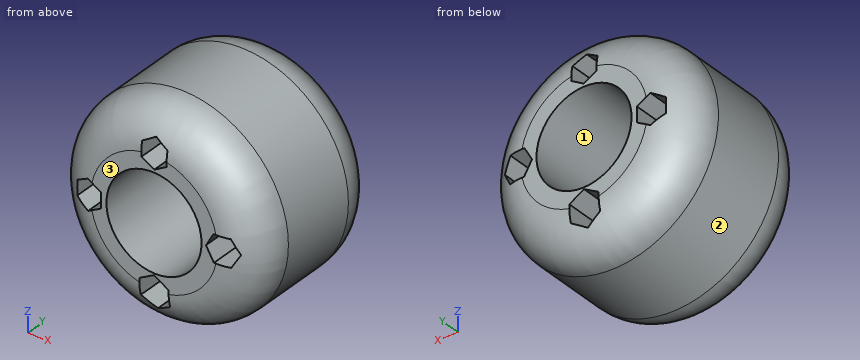
```python
from build123d import *

# Parameters (mm, degrees)
F0_R     = 5
F0_R_2   = 2.3
F1_DEPTH = 3.8


# Not quite as in the source:
# - a fillet or chamfer that OpenCascade refuses, or shapes differently, is made with other operations: its cross-section is extruded or revolved along the edge and cut away or added


with BuildPart() as f1:
    # F0 (on Front) → F1 (new body, symmetric)
    with BuildSketch(Plane.XZ):
        Circle(F0_R)
        Polygon((0, -4.0174636819), (-0.7082950324, -3.6085293543), (-0.7082950324, -2.7906606991), (0, -2.3817263714), (0.7082950324, -2.7906606991), (0.7082950324, -3.6085293543), align=None, mode=Mode.SUBTRACT)
        Polygon((-3.1964122335, 0.7368465077), (-2.5582844391, 0.3684232539), (-2.5582844391, -0.3684232539), (-3.1964122335, -0.7368465077), (-3.8345400279, -0.3684232539), (-3.8345400279, 0.3684232539), align=None, mode=Mode.SUBTRACT)
        Circle(F0_R_2, mode=Mode.SUBTRACT)
        Polygon((2.8982667587, -0.6579181574), (2.512562897, -0.0101405277), (2.8807028495, 0.6477776297), (3.6345466637, 0.6579181574), (4.0202505254, 0.0101405277), (3.6521105729, -0.6477776297), align=None, mode=Mode.SUBTRACT)
        Polygon((0.6046901305, 3.5066245139), (0.6168706685, 2.8013560578), (0.012180538, 2.4381731744), (-0.6046901305, 2.7802587472), (-0.6168706685, 3.4855272032), (-0.012180538, 3.8487100866), align=None, mode=Mode.SUBTRACT)
    extrude(amount=F1_DEPTH, both=True)

    # F2: fillet of radius 1.9313708499 on 3 edges, made by hand

    # F2_s1 → F2_t2 (revolve, cut)
    with BuildSketch(Plane.XY):
        with BuildLine():
            ThreePointArc((5, 1.8686291501), (4.4343145751, 3.2343145751), (3.0686291501, 3.8))
            Line((3.0686291501, 3.8), (5, 3.8))
            Line((5, 3.8), (5, 1.8686291501))
        make_face()
    revolve(axis=Axis((0, 3.8, 0), (0, -1, 0)), mode=Mode.SUBTRACT)

    # F2_s3 → F2_t4 (revolve, cut)
    with BuildSketch(Plane.XY):
        with BuildLine():
            ThreePointArc((5, -1.8686291501), (4.4343145751, -3.2343145751), (3.0686291501, -3.8))
            Line((3.0686291501, -3.8), (5, -3.8))
            Line((5, -3.8), (5, -1.8686291501))
        make_face()
    revolve(axis=Axis((0, -3.8, 0), (0, -1, 0)), mode=Mode.SUBTRACT)


solid = f1.part
```
Work out the finished part from the listing and answer in its coordinate system (mm). Face numbers are marked on the shaded views. Round coordinates to 2 decimals unless told otherwise and drop trailing zeros. Loops run counter-clockwise (first coordinate to the right, second up) from the corner with the lowest first, then second, coordinate; pieces in that order, holes last.
(1) Each of these flat-tipped pins is pushed along its axis until it touches: P1, Ø5, axis at x = 2, z = -3.5, coming from the +Y side; P2, Ø3, axis at y = 0.5, z = -3, coming from the +X side; P3, Ø2, axis at y = 2, z = -2.5, coming from the -X side; P4, Ø0.9, axis at y = -0.5, z = -3, coming from the -X side. Where does it stop, or does it pass through?
Computed values:
P1: stops at y = 3.8
P2: stops at x = 4.77
P3: stops at x = -4.77
P4: stops at x = -4.3
(2) The mould has two halves that part along X. Classify the marked faces 1, 2 and 3: pulls with the +X half, pulls with the -X half, needs draft (parallel to the pull), parting line crosses it, or undercut.
Computed values:
face 1: undercut
face 2: parting line crosses it
face 3: needs draft
(3) Find the intervals of material crossed by L1, parallel to Z at x = 1.5, y = 2.75; L2, parallel to Z at x = -3.5, y = -0.75; L3, parallel to Y at x = -2.75, z = 2.25, in increasing order.
Computed values:
L1: z = -4.55 to -1.74, 1.74 to 4.55
L2: z = -3.57 to -0.56, 0.56 to 3.57
L3: y = -3.74 to 3.74
(4) The part is cut by section B-B, the plane y = -3. Give the vertices of the cut face in (x, z), and give its area (3 significant figures).
Computed values:
outline: circle Ø9.27 at (0, 0); hole (-3.83, -0.37) - (-3.2, -0.74) - (-2.56, -0.37) - (-2.56, 0.37) - (-3.2, 0.74) - (-3.83, 0.37) - close; hole circle Ø4.6 at (0, 0); hole (-0.71, -3.61) - (0, -4.02) - (0.71, -3.61) - (0.71, -2.79) - (0, -2.38) - (-0.71, -2.79) - close; hole (-0.62, 3.49) - (-0.6, 2.78) - (0.01, 2.44) - (0.62, 2.8) - (0.6, 3.51) - (-0.01, 3.85) - close; hole (2.51, -0.01) - (2.9, -0.66) - (3.65, -0.65) - (4.02, 0.01) - (3.63, 0.66) - (2.88, 0.65) - close
area: 44.9 mm2
(5) The part is cut by section A-A, the plane y = 1. Give the vertices of the cut face in (x, z), and give its area (3 significant figures).
Computed values:
outline: circle Ø10 at (0, 0); hole (-3.83, -0.37) - (-3.2, -0.74) - (-2.56, -0.37) - (-2.56, 0.37) - (-3.2, 0.74) - (-3.83, 0.37) - close; hole circle Ø4.6 at (0, 0); hole (-0.71, -3.61) - (0, -4.02) - (0.71, -3.61) - (0.71, -2.79) - (0, -2.38) - (-0.71, -2.79) - close; hole (-0.62, 3.49) - (-0.6, 2.78) - (0.01, 2.44) - (0.62, 2.8) - (0.6, 3.51) - (-0.01, 3.85) - close; hole (2.51, -0.01) - (2.9, -0.66) - (3.65, -0.65) - (4.02, 0.01) - (3.63, 0.66) - (2.88, 0.65) - close
area: 56.0 mm2
